The listing builds one solid part. Answer for the finished solid, in the listing's coordinates (mm). A direction names the side the tool comes from. Round coordinates to 2 decimals unless told otherwise and drop trailing zeros. Write each loop counter-clockwise with the first axis right and the second up, starting at its lowest first coordinate (ties: lowest second). Pieces come first, ordered by that corner, then holes. Notation, with made-up numbers: M 87.25,27.25 L 143.25,27.25 A28 cw 143.25,50.25 Z; hole C -40,74.5 d3. An arc over 180 degrees is marked long. Put each result on its own line as item: value. Start each with the question number.
```python
from build123d import *

# Parameters (mm, degrees)
BOSS_EXTRUDE1_DEPTH      = 2.54
SKETCH2_W                = 9.525
SKETCH2_H                = 38.1
BOSS_EXTRUDE2_DEPTH      = 15.875
BOSS_EXTRUDE3_DEPTH      = 5.08
M3_CLEARANCE_HOLE1_D     = 3.3
M3_CLEARANCE_HOLE1_DEPTH = 12.7
M3_CLEARANCE_HOLE1_TIP   = 0.991420021
SKETCH7_W                = 35.71875
SKETCH7_H                = 2.38125
CUT_EXTRUDE1_DEPTH       = 2.54
FILLET1_R                = 1.27


with BuildPart() as part:
    # Sketch1 → Boss-Extrude1 (new body)
    with BuildSketch(Plane(origin=(0, 0, 0), x_dir=(1, 0, 0), z_dir=(0, 1, 0))):
        Polygon((0, 0), (38.1, 0), (38.1, 2.38125), (2.38125, 2.38125), (2.38125, 38.1), (0, 38.1), align=None)
    extrude(amount=BOSS_EXTRUDE1_DEPTH)

    # Sketch2 → Boss-Extrude2 (add)
    with BuildSketch(Plane(origin=(0, 2.54, 0), x_dir=(1, 0, 0), z_dir=(0, 1, 0))):
        with Locations((-4.7625, 19.05)):
            Rectangle(SKETCH2_W, SKETCH2_H)
        Polygon((0, 0), (-9.525, 0), (-9.525, -9.525), (38.1, -9.525), (38.1, 0), align=None)
    extrude(amount=-BOSS_EXTRUDE2_DEPTH)

    # Sketch3 → Boss-Extrude3 (add)
    with BuildSketch(Plane(origin=(0, -13.335, 0), x_dir=(-1, 0, 0), z_dir=(0, -1, 0))):
        Polygon((9.525, -9.525), (-38.1, -9.525), (-38.1, 18.373079092), (-18.373079092, 38.1), (9.525, 38.1), align=None)
    extrude(amount=BOSS_EXTRUDE3_DEPTH)

    # M3 Clearance Hole1
    with Locations(Plane(origin=(0, -18.415, 0), x_dir=(-1, 0, 0), z_dir=(0, -1, 0))):
        with Locations((-10, 32.5), (-32.5, 10)):
            Hole(M3_CLEARANCE_HOLE1_D / 2, depth=M3_CLEARANCE_HOLE1_DEPTH)
            with Locations((0, 0, -(M3_CLEARANCE_HOLE1_DEPTH + M3_CLEARANCE_HOLE1_TIP / 2))):  # 118° drill point
                Cone(0, M3_CLEARANCE_HOLE1_D / 2, M3_CLEARANCE_HOLE1_TIP, mode=Mode.SUBTRACT)

    # Sketch7 → Cut-Extrude1 (cut)
    with BuildSketch(Plane(origin=(0, 2.54, 0), x_dir=(1, 0, 0), z_dir=(0, 1, 0))):
        with Locations((20.240625, 1.190625)):
            Rectangle(SKETCH7_W, SKETCH7_H)
        Polygon((0, 0), (2.38125, 0), (2.38125, 2.38125), (2.38125, 38.1), (0, 38.1), align=None)
    extrude(amount=-CUT_EXTRUDE1_DEPTH, mode=Mode.SUBTRACT)

    # Fillet1
    fillet1_edges = [part.edges().sort_by_distance(p)[0] for p in [
        (38.1, 2.54, 4.7625),
        (0, -5.3975, -38.1),
        (-9.525, -7.9375, -38.1),
        (38.1, -5.3975, 0),
        (14.2875, 2.54, 9.525),
        (38.1, -7.9375, 9.525),
        (-9.525, -7.9375, 9.525),
        (-9.525, 2.54, -14.2875),
        (-9.525, -18.415, -14.2875),
        (14.2875, -18.415, 9.525),
        (-4.7625, 2.54, -38.1),
        (0, 2.54, -19.05),
        (19.05, 2.54, 0),
    ]]
    fillet(fillet1_edges, radius=FILLET1_R)


solid = part.part
```
Item 1: Consider line 1 along Z through (x, y) = (10, -14.6) (3 decimals); line 2 along X through (y, z) = (-14.5, -10) (3 decimals); line 3 along X through (y, z) = (-4, -33) (3 decimals). Determine where each line is inside the solid, lowest interval first. Write a range as [from, to].
Item 2: Section A-A (x = 10) is taken. Give the vertices of the cut face in (y, z) (3 decimals), and give its area (3 significant figures).
Item 3: Flat-ended cylindrical pins translate along their axes: pin 1 (7.5 mm diameter, centred on x = 12, y = -2.5, fed in from -Z); pin 2 (7.5 mm diameter, centred on y = -6, z = -19.5, fed in from +X). Find the tip coordinate at first contact, or state that the pin passes through.
Item 4: Section C-C (y = -16) is taken. Give the vertices of the cut face in (x, z) (3 decimals), and give its area (3 significant figures).
Item 5: Section D-D (x = 16.5) is taken. Give the vertices of the cut face in (y, z) (3 decimals).
Item 6: Section B-B (z = -10) is taken. Give the vertices of the cut face in (x, y) (3 decimals).
Item 7: Determine the mould class of faces 1 (the cylindrical face through (31.19, -15.84, -9)), 2 (the cylindrical face through (18.047, 2.158, 0.362)), 3 (the cylindrical face through (10.89, -15.84, -33.89)), 4 (the cylindrical face through (-9.16, 2.16, -13.97)) for opening direction X: released by +X, released by -X, zero draft, split by the parting line, or undercut.
Item 8: Which of the six approach directions +Z, -Z, +X, -X, +Y, -Y give full straight-line access (tool end or side, diameter ignored) to faces 5 (the flat face through (-1, -15, -38.1)), 6 (the cylindrical face through (37.718, -5.93, 0.362))?
Output values:
1. line 1: z = [-38.1, -34.15], [-30.85, 9.525]
1. line 2: x = [-9.525, 30.85], [34.15, 38.1]
1. line 3: x = [-9.525, 0]
2. outline: M -18.415,-38.1 L -13.335,-38.1 L -13.335,-34.15 L -18.415,-34.15 Z; M -18.415,-30.85 L -13.335,-30.85 L -13.335,0 L 1.27,0 A1.27 ccw 2.54,1.27 L 2.54,8.255 A1.27 ccw 1.27,9.525 L -17.145,9.525 A1.27 ccw -18.415,8.255 Z
2. area: 375 mm^2
3. pin 1: stops at z = 0
3. pin 2: stops at x = 0
4. outline: M -9.525,-36.83 A1.27 ccw -8.255,-38.1 L 18.373,-38.1 L 38.1,-18.373 L 38.1,8.255 A1.27 ccw 36.83,9.525 L -8.255,9.525 A1.27 ccw -9.525,8.255 Z; hole C 10,-32.5 d3.3; hole C 32.5,-10 d3.3
4. area: 2,060 mm^2
5. outline: M -18.415,-38.1 L -13.335,-38.1 L -13.335,0 L 1.27,0 A1.27 ccw 2.54,1.27 L 2.54,8.255 A1.27 ccw 1.27,9.525 L -17.145,9.525 A1.27 ccw -18.415,8.255 Z
6. outline: M -9.525,-17.145 A1.27 ccw -8.255,-18.415 L 30.85,-18.415 L 30.85,-13.335 L 0,-13.335 L 0,1.27 A1.27 ccw -1.27,2.54 L -8.255,2.54 A1.27 ccw -9.525,1.27 Z; M 34.15,-18.415 L 38.1,-18.415 L 38.1,-13.335 L 34.15,-13.335 Z
7. face 1: undercut
7. face 2: zero draft
7. face 3: undercut
7. face 4: released by -X
8. face 5: -Z, +X, -X, +Y, -Y
8. face 6: -Z, +X, +Y
